Work out the finished part from the listing and answer in its coordinate system (mm). A direction names the side the tool comes from. Give positions to 0.01 mm unless a question says otherwise; leave off trailing zeros. Write each loop counter-clockwise with the first axis right and the second up, starting at its lowest first coordinate (ties: lowest second). Pieces come first, ordered by that corner, then holes. Notation, with made-up numbers: (-4.5, 56) - (13.5, 56) arc R25 ccw to (13.5, 82) - close; hole circle Ø6 at (80, -35). An arc over 180 degrees is marked (long way). Write item = value, one per line.
from build123d import *

# Parameters (mm, degrees)
SKETCH1_R           = 12.7
BOSS_EXTRUDE1_DEPTH = 3
BOSS_EXTRUDE2_DEPTH = 12.7
CUT_EXTRUDE1_DEPTH  = 23


with BuildPart() as part:
    # Sketch1 → Boss-Extrude1 (new body)
    with BuildSketch(Plane(origin=(0, 0, 0), x_dir=(1, 0, 0), z_dir=(0, 1, 0))):
        with Locations(Location((0, 0, 0), (0, 0, 270))):
            Circle(SKETCH1_R)
    extrude(amount=BOSS_EXTRUDE1_DEPTH)

    # Sketch2 → Boss-Extrude2 (add)
    with BuildSketch(Plane(origin=(0, 3, 0), x_dir=(1, 0, 0), z_dir=(0, 1, 0))):
        Polygon((0.148889151, -5.48), (4.820263788, -2.611058213), (4.671374637, 2.868941787), (-0.148889151, 5.48), (-4.820263788, 2.611058213), (-4.671374637, -2.868941787), align=None)
    extrude(amount=BOSS_EXTRUDE2_DEPTH)

    # Sketch6 → Cut-Extrude1 (cut)
    with BuildSketch(Plane(origin=(0, 15.7, 0), x_dir=(1, 0, 0), z_dir=(0, 1, 0))):
        Polygon((-2.597868549, -1.386029942), (-0.098597134, -2.94283513), (2.499271415, -1.556805188), (2.597868549, 1.386029942), (0.098597134, 2.94283513), (-2.499271415, 1.556805188), align=None)
    extrude(amount=-CUT_EXTRUDE1_DEPTH, mode=Mode.SUBTRACT)


solid = part.part
1. Find section D-D, the plane x = 3.5. Give the vertices of the cut face in (y, z).
Solution:
outline = (0, -12.21) - (3, -12.21) - (3, -3.5) - (15.7, -3.5) - (15.7, 3.42) - (3, 3.42) - (3, 12.21) - (0, 12.21) - close
2. A tool of negligible diameter and unlimited length cuts with its end or side. For faces 1 (the flat face through (1.18, 7.96, 2.26)), 2 (the flat face through (-5, 3, 0)), 3 (the flat face through (-2.29, 9.26, 4.16)), 4 (the flat face through (2.29, 9.26, -4.16)), from which of +Z, -Z, +X, -X, +Y, -Y can it reach the whole face along a straight path? Write none if from no direction.
Solution:
face_1 = +Y, -Y
face_2 = +Y
face_3 = +Z, -X, +Y
face_4 = -Z, +X, +Y
3. Find section B-B, the plane z = 0.75. Give the vertices of the cut face in (x, y).
Solution:
outline = (-12.68, 0) - (-2.58, 0) - (-2.58, 15.7) - (-4.73, 15.7) - (-4.73, 3) - (-12.68, 3) - close; (2.53, 0) - (12.68, 0) - (12.68, 3) - (4.77, 3) - (4.77, 15.7) - (2.53, 15.7) - close
4. Find section C-C, the plane y = 10.5. Give the vertices of the cut face in (x, z), then the cut area to 3 significant figures.
Solution:
outline = (-4.82, -2.61) - (-0.15, -5.48) - (4.67, -2.87) - (4.82, 2.61) - (0.15, 5.48) - (-4.67, 2.87) - close; hole (-2.6, 1.39) - (-2.5, -1.56) - (0.1, -2.94) - (2.6, -1.39) - (2.5, 1.56) - (-0.1, 2.94) - close
area = 55.6 mm^2
5. Given pin 1 (1 mm diameter, centred on x = 9.5, z = 5.5, fed in from +Y); pin 2 (1 mm diameter, centred on x = -6, y = 10, fed in from +Z); pin 3 (3 mm diameter, centred on x = 8.5, y = 1.5, fed in from +Z); pin 4 (1 mm diameter, centred on y = 13.5, z = -0.5, fed in from -X), each flat-ended and moving along its own axis, determine where each tip first touches the part or whether it passes through.
Solution:
pin_1 = 3
pin_2 = through
pin_3 = 10.6
pin_4 = -4.78
6. Find section A-A, the plane y = 2.25. Give the vertices of the cut face in (x, z).
Solution:
outline = circle Ø25.4 at (0, 0); hole (-2.6, 1.39) - (-2.5, -1.56) - (0.1, -2.94) - (2.6, -1.39) - (2.5, 1.56) - (-0.1, 2.94) - close
7. For a pull along X with two mould halves and no side action, classify faces 5 (the flat face through (2.452, 9.261, 4.066)), 6 (the flat face through (-1.37, 7.96, 2.15)), 7 (the flat face through (-2.452, 9.261, -4.066)) as pulls with the +X half, pulls with the -X half, needs draft (parallel to the pull), parting line crosses it, or undercut.
Solution:
face_5 = pulls with the +X half
face_6 = undercut
face_7 = pulls with the -X half
8. Straight lines are drawn through the part: line 1 (Y direction, x = 9.5, z = 2.25); line 2 (Z direction, x = -0.5, y = 7); line 3 (Z direction, x = 1, y = 4.75). For each, find the intervals that lie inside material, in ascending order.
Solution:
line_1 = 0 to 3
line_2 = -5.26 to -2.62, 2.69 to 5.13
line_3 = -4.86 to -2.38, 2.36 to 4.96
